Autodesk Inventor part; units mm, degrees
ref_plane "Start Plane" through (0, 0, -4.9897) normal (0, 0, 1) x (1, 0, 0)
ref_plane "End Plane" through (0, 0, 247.019) normal (0, 0, 1) x (1, 0, 0)
ref_plane "Work Plane4" through (0.3845, -10.6611, 247.658) normal (-0.0193, 0.5358, 0.8441) x (0.9998, 0.0056, 0.0193)
ref_plane "Start Plane" through (0, 0, -4.9897) normal (0, 0, 1) x (1, 0, 0)
ref_plane "End Plane" through (0, 0, 247.019) normal (0, 0, 1) x (1, 0, 0)
sketch "Sketch" plane through (0, 0, 0) normal (0, 0, 1) x (1, 0, 0)
  circle A0 centre (0, 0) radius 6.9342
  circle A1 centre (0, 0) radius 10.668
  dimension "d0" = 21.336
  dimension "d1" = 3.7338
extrude "Body" add sketch "Sketch" along normal up to surface (252.0086 mm away) from surface at -4.9897
sketch "Sketch3" plane through (0, 0, 0) normal (0, 0, 1) x (1, 0, 0)
  line L0 (0, 0) -> (10, 0)
ref_plane "Work Plane3" through (0, 0, 0) normal (0, -1, 0) x (1, 0, 0)
sketch "Sketch4" plane through (0, 0, 0) normal (0, -1, 0) x (1, 0, 0)
  line L0 (-2, -4.9897) -> (12, -4.9897)
  line L1 (-2, 247.019) -> (12, 247.019)
  dimension "d7" = 252.0086
ref_plane "Work Plane4" through (0.3845, -10.6611, 247.658) normal (-0.0193, 0.5358, 0.8441) x (0.9998, 0.0056, 0.0193)
split "Split1" plane through (0.3845, -10.6611, 247.658) removes the side toward (-0.0193, 0.5358, 0.8441)
ref_plane "Work Plane5" through (8.2715, -6.7371, 260.0533) normal (-0.6775, 0.5518, 0.4862) x (0.6911, 0.2516, 0.6775)
split "Split2" plane through (8.2715, -6.7371, 260.0533) removes the side toward (-0.6775, 0.5518, 0.4862)
ref_plane "Work Plane6" through (-10.464, -2.0762, 252.5557) normal (0.7241, 0.1437, 0.6746) x (0.6869, -0.0621, -0.7241)
split "Split3" plane through (-10.464, -2.0762, 252.5557) removes the side toward (0.7241, 0.1437, 0.6746)
ref_plane "Work Plane7" through (4.2865, -9.7689, -6.8509) normal (-0.2171, 0.4948, -0.8414) x (0.7027, 0.6776, 0.2171)
split "Split4" plane through (4.2865, -9.7689, -6.8509) removes the side toward (-0.2171, 0.4948, -0.8414)
ref_plane "Work Plane8" through (-10.464, -2.0762, -9.7489) normal (0.6617, 0.1313, -0.7382) x (-0.6724, -0.3318, -0.6617)
split "Split5" plane through (-10.464, -2.0762, -9.7489) removes the side toward (0.6617, 0.1313, -0.7382)
equation "\"d0\" = G_H"
equation "\"d1\" = G_T"
equation "\"d2\" = G_L"
equation "\"G_H\" = 21.336"
equation "\"G_T\" = 3.7338"
equation "\"G_L\" = 252.00863"
equation "\"G_OFFSET_START\" = 4.98966"
equation "\"G_OFFSET_END\" = 6.137"
equation "\"d4\" = -G_OFFSET_START"
equation "\"d5\" = G_OFFSET_END + B_L"
equation "\"B_L\" = 240.88196"
properties part number "ANSI - 1/2 x 0.147 - 9.922" material "Steel, Mild"
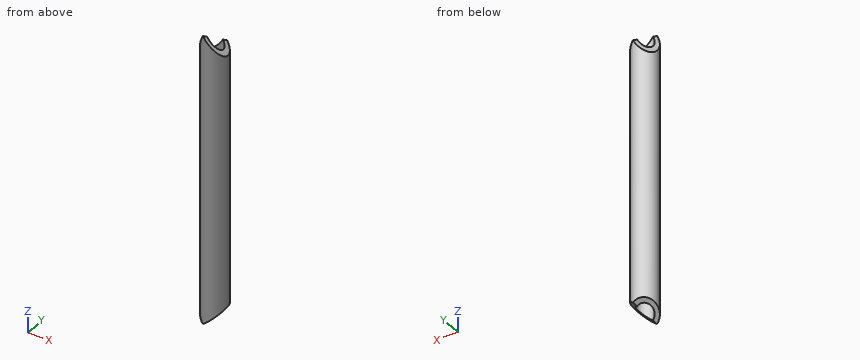
Source: CAD feature listing. Evaluate the final solid. Frame: model axes, mm. Round coordinates to 2 decimals unless told otherwise and drop trailing zeros. Loops run counter-clockwise (first coordinate to the right, second up) from the corner with the lowest first, then second, coordinate; pieces in that order, holes last.
1. Contact query for flat-ended pins moving along their axis: pin 1 (8.5 mm diameter, centred on x = 0, y = 0, fed in from +Z); pin 2 (12 mm diameter, centred on x = 7, z = 59.5, fed in from -Y); pin 3 (4 mm diameter, centred on y = 4, z = 57.5, fed in from +X); pin 4 (5 mm diameter, centred on y = -6.5, z = 81, fed in from +X). Output: stop coordinate, or through.
2. Section query A-A on x = 0. Output: boundary loops of the cut face in (y, z), and give its area (3 significant figures).
3. Section query B-B on z = 61. Output: boundary loops of the cut face in (x, y), and give its area (3 significant figures).
4. Ray query, L1, parallel to X at y = 0, z = 81; L2, parallel to X at y = 4.75, z = 43.5. Return the intervals inside material, ascending.
5. Section query C-C on y = 0. Output: boundary loops of the cut face in (x, z), and give its area (3 significant figures).
Answers below:
1. pin 1: passes through
1. pin 2: stops at y = -10.62
1. pin 3: stops at x = 10.48
1. pin 4: stops at x = 9.89
2. outline: (-10.67, -1.9) - (-6.93, -1.23) - (-6.93, 242.36) - (-10.67, 243.15) - close; (6.93, 4.08) - (10.67, 6.27) - (10.67, 228.77) - (6.93, 233.01) - close
2. area: 1,760 mm2
3. outline: circle Ø21.34 at (0, 0); hole circle Ø13.87 at (0, 0)
3. area: 206 mm2
4. L1: x = -10.67 to -6.93, 6.93 to 10.67
4. L2: x = -9.55 to -5.05, 5.05 to 9.55
5. outline: (-10.67, 2.75) - (-6.93, 1.79) - (-6.93, 231.22) - (-10.67, 226.02) - close; (6.93, 6.22) - (10.67, 9.56) - (10.67, 229.43) - (6.93, 233.44) - close
5. area: 1,680 mm2
